The model under review builds one solid part; all positions refer to its coordinate system, in mm. A direction names the side the tool comes from. Give positions to 0.01 mm unless a question says otherwise; leave off trailing zeros. Order: outer loops, then holes, each group sorted by start corner. A loop starts at its lowest first (then second) coordinate and runs counter-clockwise, first axis right, second up. Notation, with made-up numbers: (-13, -23.75) - (41, -23.75) arc R12 cw to (41, -12.75) - close; hole circle Ø2 at (25, -24.75). An arc over 180 degrees is marked (long way). Use CSV: the item, a comma, the result in double quotes.
```python
from build123d import *

# Parameters (mm, degrees)
F0_W      = 15.3
F0_H      = 31
F1_DEPTH  = 1
F2_DEPTH  = 5
F3_W      = 1.9
F3_H      = 2.1
F3_H_2    = 0.4
F4_DEPTH  = 2.6
F5_W      = 1.9
F5_H      = 2
F6_DEPTH  = 2.1
F7_W      = 19.3
F7_H      = 5
F8_DEPTH  = 50
F9_SIZE   = 2
F10_DEPTH = 25
F11_W     = 10
F11_H     = 10
F11_R     = 1.75
F12_DEPTH = 5


with BuildPart() as f1:
    # F0 (on Front) → F1 (new body)
    with BuildSketch(Plane.XZ):
        with Locations((0.723570025, -27.1247635409)):
            Rectangle(F0_W, F0_H)
    extrude(amount=F1_DEPTH)

    # F0 (on Front) → F2 (join)
    with BuildSketch(Plane.XZ):
        Polygon((-6.926429975, -42.6247635409), (-6.926429975, -11.6247635409), (-8.926429975, -11.6247635409), (-8.926429975, -44.6247635409), (10.373570025, -44.6247635409), (10.373570025, -11.6247635409), (8.373570025, -11.6247635409), (8.373570025, -42.6247635409), align=None)
    extrude(amount=F2_DEPTH)

    # F3 (on face) → F4 (join)
    with BuildSketch(Plane.XY.offset(-42.6247635409)):
        with Locations((-5.976429975, -6.05)):
            Rectangle(F3_W, F3_H)
        with Locations((-5.976429975, -4.8)):
            Rectangle(F3_W, F3_H_2)
        with Locations((7.423570025, -6.05)):
            Rectangle(F3_W, F3_H)
        with Locations((7.423570025, -4.8)):
            Rectangle(F3_W, F3_H_2)
    extrude(amount=F4_DEPTH)

    # F5 (on face) → F6 (join)
    with BuildSketch(Plane.XZ.offset(5)):
        with Locations((-5.976429975, -43.6247635409)):
            Rectangle(F5_W, F5_H)
        with Locations((7.423570025, -43.6247635409)):
            Rectangle(F5_W, F5_H)
    extrude(amount=F6_DEPTH)

    # F7 (on face) → F8 (join)
    with BuildSketch(Plane(origin=(0, 0, -44.6247635409), x_dir=(1, 0, 0), z_dir=(0, 0, -1))):
        with Locations((0.723570025, -2.5)):
            Rectangle(F7_W, F7_H)
        Polygon((-6.926429975, 5), (-8.926429975, 5), (-8.926429975, 0), (10.373570025, 0), (10.373570025, 5), (8.373570025, 5), (6.473570025, 5), (-5.026429975, 5), align=None)
    extrude(amount=F8_DEPTH)

    # F9
    f9_edges = [f1.edges().sort_by_distance(p)[0] for p in [
        (7.42357, -7.1, -44.624764),
        (-5.97643, -7.1, -44.624764),
    ]]
    chamfer(f9_edges, length=F9_SIZE)

    # F10 (add): a face of the model
    f10_faces = [f1.faces().sort_by_distance(p)[0] for p in [
        (0.723570025, 2.5, -44.6247635409),
    ]]
    extrude(f10_faces, amount=F10_DEPTH)

    # F11 (on face) → F12 (join)
    with BuildSketch(Plane(origin=(0, 0, -94.6247635409), x_dir=(1, 0, 0), z_dir=(0, 0, -1))):
        with Locations((15.373570025, 0)):
            Rectangle(F11_W, F11_H)
        with Locations((15.373570025, 0)):
            Circle(F11_R, mode=Mode.SUBTRACT)
    extrude(amount=-F12_DEPTH)


solid = f1.part
```
Item 1: Take a section at B-B, the plane y = 1. Give the boundary of the cut face in (x, z).
Results list:
outline,"(-8.93, -94.62) - (13.94, -94.62) - (13.94, -89.62) - (10.37, -89.62) - (10.37, -19.62) - (-8.93, -19.62) - close; (16.81, -94.62) - (20.37, -94.62) - (20.37, -89.62) - (16.81, -89.62) - close"
Item 2: Wall thickness on L1, parallel to X at y = 0, z = -90.9; L2, parallel to Z at x = -0.5, y = 4; L3, parallel to Y at x = -6.75, z = -17: over which ranges is each line inside the solid? List them lowest first.
Results list:
L1,"x = -8.93 to 13.62, 17.12 to 20.37"
L2,"z = -94.62 to -19.62"
L3,"y = -1 to 0"
Item 3: Take a section at D-D, the plane x = 15. Give the boundary of the cut face in (y, z).
Results list:
outline,"(-5, -94.62) - (-1.71, -94.62) - (-1.71, -89.62) - (-5, -89.62) - close; (1.71, -94.62) - (5, -94.62) - (5, -89.62) - (1.71, -89.62) - close"
Item 4: Take a section at C-C, the plane z = -37. Give the boundary of the cut face in (x, y), and give its area (3 significant figures).
Results list:
outline,"(-8.93, -5) - (-6.93, -5) - (-6.93, -1) - (8.37, -1) - (8.37, -5) - (10.37, -5) - (10.37, 5) - (-8.93, 5) - close"
area,"132 mm2"
Item 5: Clearance check with flat-ended pins moving along their axes: pin 1 (0.6 mm diameter, centred on x = -6.5, y = -6, fed in from +Z); pin 2 (9 mm diameter, centred on x = 1.5, z = -69.5, fed in from -Y); pin 3 (1.5 mm diameter, centred on x = -0.5, y = 1.5, fed in from +Z); pin 4 (3 mm diameter, centred on x = 15.37, y = 0, fed in from -Z). State where each tip first meets the part, or that it passes through.
Results list:
pin 1,"stops at z = -40.02"
pin 2,"stops at y = -5"
pin 3,"stops at z = -19.62"
pin 4,"passes through"
Item 6: Take a section at A-A, the plane x = 4.5. Give the boundary of the cut face in (y, z).
Results list:
outline,"(-5, -94.62) - (5, -94.62) - (5, -19.62) - (0, -19.62) - (0, -11.62) - (-1, -11.62) - (-1, -42.62) - (-5, -42.62) - close"
Item 7: Mouldability with a two-part tool opening along Y and no side actions: class faces 4 (the face through (10.374, 0, -51)), 5 (the face through (1, -3, -42.625)), 6 (the face through (7.41, -6.086, -43.639)) as pulls with the +Y half, pulls with the -Y half, needs draft (parallel to the pull), parting line crosses it, or undercut.
Results list:
face 4,"needs draft"
face 5,"undercut"
face 6,"pulls with the -Y half"
Item 8: Tool access review of faces 1 (the face through (-6, -4.6, -41)), 2 (the face through (-6, -6, -40.025)), 3 (the face through (8.374, -6, -42)): name each direction out of +Z, -Z, +X, -X, +Y, -Y from which nothing blocks a thin tool from reaching the whole face with its end or side.
Results list:
face 1,"+Z"
face 2,"+Z, -Y"
face 3,"+Z, -Z, +X, -Y"
